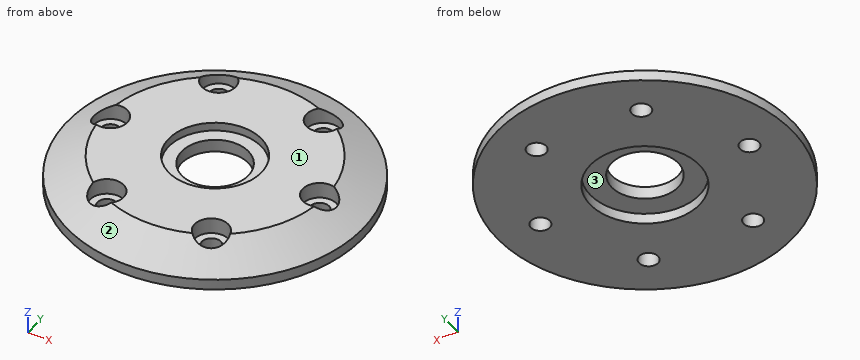
```python
from build123d import *

# Parameters (mm, degrees)
SKETCH1_R               = 35
BOSS_EXTRUDE1_DEPTH     = 5
BOSS_EXTRUDE1_TAPER     = 60
SKETCH3_R               = 11
CUT_EXTRUDE1_DEPTH      = 2
SKETCH4_R               = 7.9
CUT_EXTRUDE2_DEPTH      = 81.661329025
SKETCH7_R               = 35
SKETCH7_R_2             = 12.95
BOSS_EXTRUDE2_DEPTH     = 2.5
CUT_EXTRUDE6_DEPTH      = 81.661329025
CUT_EXTRUDE6_DEPTH_BACK = 81.661329025
SKETCH5_R               = 2.25
SKETCH8_R               = 4
CUT_EXTRUDE8_DEPTH      = 3.75


with BuildPart() as part:
    # Sketch1 → Boss-Extrude1 (new body)
    with BuildSketch(Plane.XY):
        with Locations((0, 37.5)):
            Circle(SKETCH1_R)
    extrude(amount=BOSS_EXTRUDE1_DEPTH, taper=BOSS_EXTRUDE1_TAPER)

    # Sketch3 → Cut-Extrude1 (cut)
    with BuildSketch(Plane.XY.offset(5)):
        with Locations((0, 37.5)):
            Circle(SKETCH3_R)
    extrude(amount=-CUT_EXTRUDE1_DEPTH, mode=Mode.SUBTRACT)

    # Sketch4 → Cut-Extrude2 (cut, through all)
    with BuildSketch(Plane.XY.offset(5)):
        with Locations((0, 37.5)):
            Circle(SKETCH4_R)
    extrude(amount=-CUT_EXTRUDE2_DEPTH, mode=Mode.SUBTRACT)

    # Sketch7 → Boss-Extrude2 (add)
    with BuildSketch(Plane.XY):
        with Locations((0, 37.5)):
            Circle(SKETCH7_R)
        with Locations((0, 37.5)):
            Circle(SKETCH7_R_2, mode=Mode.SUBTRACT)
    extrude(amount=-BOSS_EXTRUDE2_DEPTH)

    # Sketch5 → Cut-Extrude6 (cut, two sides: drawn at the far end of the back side and taken through both)
    with BuildSketch(Plane.XY.offset(-CUT_EXTRUDE6_DEPTH_BACK)):
        with Locations(Location((-12.5, 15.849364905, 0), (0, 0, 184.499391781))):
            Circle(SKETCH5_R)
        with Locations(Location((-25, 37.5, 0), (0, 0, 124.499391764))):
            Circle(SKETCH5_R)
        with Locations(Location((-12.5, 59.150635095, 0), (0, 0, 175.50060828))):
            Circle(SKETCH5_R)
        with Locations(Location((12.5, 59.150635095, 0), (0, 0, 115.50060828))):
            Circle(SKETCH5_R)
        with Locations((25, 37.5)):
            Circle(SKETCH5_R)
        with Locations(Location((12.5, 15.849364905, 0), (0, 0, 244.499391764))):
            Circle(SKETCH5_R)
    extrude(amount=CUT_EXTRUDE6_DEPTH + CUT_EXTRUDE6_DEPTH_BACK, mode=Mode.SUBTRACT)

    # Sketch8 → Cut-Extrude8 (cut)
    with BuildSketch(Plane.XY.offset(5)):
        with Locations((-12.5, 59.150635095)):
            Circle(SKETCH8_R)
        with Locations((-25, 37.5)):
            Circle(SKETCH8_R)
        with Locations((12.5, 59.150635095)):
            Circle(SKETCH8_R)
        with Locations((25, 37.5)):
            Circle(SKETCH8_R)
        with Locations((12.5, 15.849364905)):
            Circle(SKETCH8_R)
        with Locations((-12.5, 15.849364905)):
            Circle(SKETCH8_R)
    extrude(amount=-CUT_EXTRUDE8_DEPTH, mode=Mode.SUBTRACT)


solid = part.part
```
Can you work these out from the model? Positions are in its coordinate system, mm. Face numbers are marked on the shaded views. Round coordinates to 2 decimals unless told otherwise and drop trailing zeros. Return JSON: item names as keys, results as strings. Group by question number.
1. If we section it at A-A, the plane y = 37.5: Count the separate pieces of the cut face and the enclosed holes in it, then the cut area to 3 significant figures.
2. I need wall thicknesses on line 1 (Y direction, x = 12.5, z = 3.5); line 2 (Y direction, x = 12.5, z = 2.15); line 3 (X direction, y = 37, z = -1.25). Which ranges of each line are inside material? Lowest first, please. Write a range as [from, to].
3. We'd pull the mould along Y, two halves only. Please class the marked faces 1, 2 and 3: released by +Y, released by -Y, zero draft, split by the parting line, or undercut.
4. Will these pins go through, and if not, where does the flat tip stop? pin 1 (1.5 mm diameter, centred on x = 11.5, z = 1, fed in from +Y); pin 2 (5 mm diameter, centred on x = -12.5, y = 59.15, fed in from +Z); pin 3 (13 mm diameter, centred on x = -5, y = 41, fed in from -Z).
Output values:
{
 "1": {"separate pieces": "4", "enclosed holes": "0", "area": "236 mm²"},
 "2": {"line 1": "[11.4, 11.85], [19.85, 55.15], [63.15, 63.6]", "line 2": "[8.83, 11.85], [19.85, 55.15], [63.15, 66.17]", "line 3": "[-35, -27.19], [-22.81, -12.94], [12.94, 22.81], [27.19, 35]"},
 "3": {"face 1": "zero draft", "face 2": "split by the parting line", "face 3": "undercut"},
 "4": {"pin 1": "y = 70.12", "pin 2": "z = 1.25", "pin 3": "z = 0"}
}
